Answer from the drawing. Dimensions are ordinates in mm from the lowest x, y and z of the part. A direction names the side the tool comes from. Coordinates: 2 decimals unless noted, no trailing zeros. Order: outer loops, then holes, each group sorted by start corner. A loop starts at its lowest first (then second) coordinate and runs counter-clockwise, first axis right, second up. Notation, with made-up numbers: (33, -13.75) - (90, -13.75) arc R13 cw to (90, -5.75) - close; hole circle Ø8 at (-34.5, -32). An arc over 180 degrees is marked (long way). Answer as a JSON object with one key per item and string values. Group by question number.
1) Find the intervals of material crossed by line 1 along Z through (x, y) = (22.5, 42.5); line 2 along X through (y, z) = (18, 6.5); line 3 along Y through (x, z) = (25.4, 24.3), in increasing order.
2) Section B-B (x = 25.4) is taken. Give the vertices of the cut face in (y, z), plus the area to 3 significant figures.
3) Section D-D (y = 12.7) is taken. Give the vertices of the cut face in (x, z).
4) The mould has two halves that part along Z. Classify the marked faces 1, 2 and 3: released by +Z, released by -Z, zero draft, split by the parting line, or undercut.
5) A tool of negligible diameter and unlimited length cuts with its end or side. For the marked faces 4 and 5, from which of +Z, -Z, +X, -X, +Y, -Y can it reach the whole face along a straight path? Write none if from no direction.
6) Section A-A (y = 57.15) is taken. Give the vertices of the cut face in (x, z), plus the area to 3 significant figures.
7) Section C-C (z = 5.5) is taken. Give the vertices of the cut face in (x, y).
8) This flat-tipped pin is pushed along its axis until it touches: P1, Ø5.5, axis at x = 9.525, y = 12.7, coming from the +Z side. Where does it stop, or does it pass through?
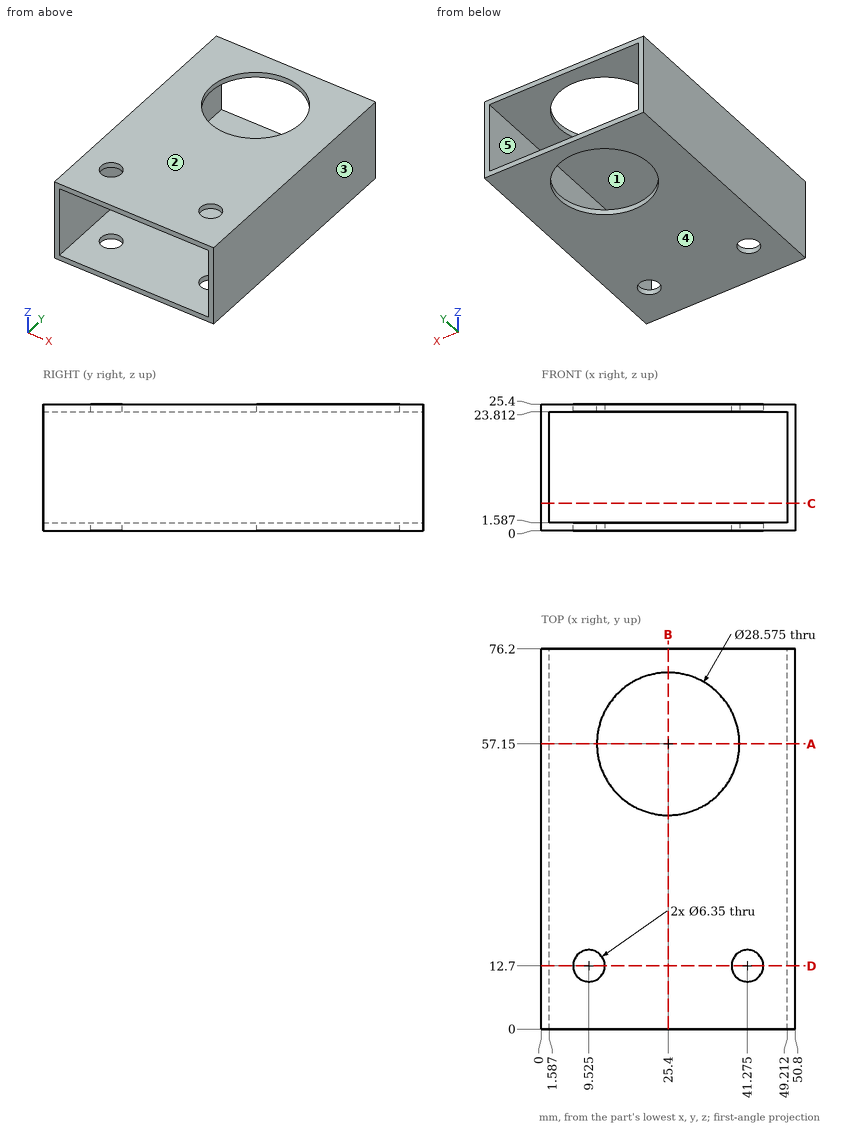
Report:
{
 "1": {"line 1": "z = 0 to 1.59, 23.81 to 25.4", "line 2": "x = 0 to 1.59, 49.21 to 50.8", "line 3": "y = 0 to 42.86, 71.44 to 76.2"},
 "2": {"outline": "(0, 0) - (42.86, 0) - (42.86, 1.59) - (0, 1.59) - close; (0, 23.81) - (42.86, 23.81) - (42.86, 25.4) - (0, 25.4) - close; (71.44, 0) - (76.2, 0) - (76.2, 1.59) - (71.44, 1.59) - close; (71.44, 23.81) - (76.2, 23.81) - (76.2, 25.4) - (71.44, 25.4) - close", "area": "151 mm²"},
 "3": {"outline": "(0, 0) - (6.35, 0) - (6.35, 1.59) - (1.59, 1.59) - (1.59, 23.81) - (6.35, 23.81) - (6.35, 25.4) - (0, 25.4) - close; (12.7, 0) - (38.1, 0) - (38.1, 1.59) - (12.7, 1.59) - close; (12.7, 23.81) - (38.1, 23.81) - (38.1, 25.4) - (12.7, 25.4) - close; (44.45, 0) - (50.8, 0) - (50.8, 25.4) - (44.45, 25.4) - (44.45, 23.81) - (49.21, 23.81) - (49.21, 1.59) - (44.45, 1.59) - close"},
 "4": {"face 1": "undercut", "face 2": "released by +Z", "face 3": "zero draft"},
 "5": {"face 4": "-Z, +X, -X, +Y, -Y", "face 5": "+Y, -Y"},
 "6": {"outline": "(0, 0) - (11.11, 0) - (11.11, 1.59) - (1.59, 1.59) - (1.59, 23.81) - (11.11, 23.81) - (11.11, 25.4) - (0, 25.4) - close; (39.69, 0) - (50.8, 0) - (50.8, 25.4) - (39.69, 25.4) - (39.69, 23.81) - (49.21, 23.81) - (49.21, 1.59) - (39.69, 1.59) - close", "area": "141 mm²"},
 "7": {"outline": "(0, 0) - (1.59, 0) - (1.59, 76.2) - (0, 76.2) - close; (49.21, 0) - (50.8, 0) - (50.8, 76.2) - (49.21, 76.2) - close"},
 "8": {"P1": "passes through"}
}
